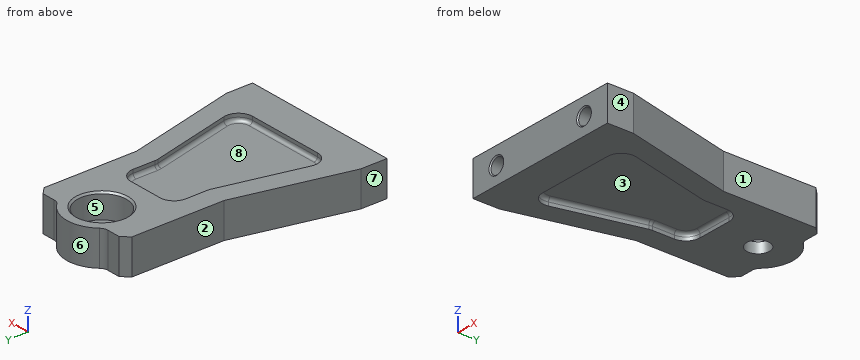
```python
from build123d import *

# Parameters (mm, degrees)
SKETCH1_R                         = 6.5
BOSS_EXTRUDE1_DEPTH               = 10
SKETCH2_R                         = 14
CUT_EXTRUDE1_DEPTH                = 14
CHAMFER1_SIZE                     = 1
CHAMFER2_SIZE                     = 4
FILLET1_R                         = 5
CUT_EXTRUDE2_DEPTH                = 4
FILLET2_R                         = 2
FILLET2_OF_MIRROR1_R              = 2
M10X1_25_TAPPED_HOLE2_D           = 8.8
M10X1_25_TAPPED_HOLE2_DEPTH       = 20
M10X1_25_TAPPED_HOLE2_CSINK_D     = 10.05
M10X1_25_TAPPED_HOLE2_CSINK_ANGLE = 90
M10X1_25_TAPPED_HOLE2_TIP         = 2.643786724


with BuildPart() as part:
    # Sketch1 → Boss-Extrude1 (new, symmetric)
    with BuildSketch(Plane.XY):
        with BuildLine():
            Line((-46, 0), (46, 0))
            Line((46, 0), (46, 15))
            Line((46, 15), (30, 80))
            Line((30, 80), (30, 137))
            Line((30, 137), (16, 137))
            ThreePointArc((16, 137), (0, 145), (-16, 137))
            Line((-16, 137), (-30, 137))
            Line((-30, 137), (-30, 80))
            Line((-30, 80), (-46, 15))
            Line((-46, 15), (-46, 0))
        make_face()
        with Locations((0, 125)):
            Circle(SKETCH1_R, mode=Mode.SUBTRACT)
    extrude(amount=BOSS_EXTRUDE1_DEPTH, both=True)

    # Sketch2 → Cut-Extrude1 (cut)
    with BuildSketch(Plane.XY.offset(10)):
        with Locations((0, 125)):
            Circle(SKETCH2_R)
    extrude(amount=-CUT_EXTRUDE1_DEPTH, mode=Mode.SUBTRACT)

    # Chamfer1
    chamfer1_edges = [part.edges().sort_by_distance(p)[0] for p in [
        (-14, 125, 10),
    ]]
    chamfer(chamfer1_edges, length=CHAMFER1_SIZE)

    # Chamfer2
    chamfer2_edges = [part.edges().sort_by_distance(p)[0] for p in [
        (-30, 137, 0),
        (30, 137, 0),
    ]]
    chamfer(chamfer2_edges, length=CHAMFER2_SIZE)

    # Fillet1
    fillet1_edges = [part.edges().sort_by_distance(p)[0] for p in [
        (-16, 137, 0),
        (16, 137, 0),
    ]]
    fillet(fillet1_edges, radius=FILLET1_R)

    # Sketch3 → Cut-Extrude2 (cut)
    with BuildSketch(Plane.XY.offset(10)):
        with BuildLine():
            Line((-18, 92), (-18, 79.514932029))
            ThreePointArc((-18, 79.514932029), (-18.058181812, 78.55185162), (-18.231880969, 77.602779652))
            Line((-18.231880969, 77.602779652), (-29.971112298, 29.912152377))
            ThreePointArc((-29.971112298, 29.912152377), (-28.49970745, 23.065287193), (-22.202993266, 20))
            Line((-22.202993266, 20), (22.202993266, 20))
            ThreePointArc((22.202993266, 20), (28.49970745, 23.065287193), (29.971112298, 29.912152377))
            Line((29.971112298, 29.912152377), (18.231880969, 77.602779652))
            ThreePointArc((18.231880969, 77.602779652), (18.058181812, 78.55185162), (18, 79.514932029))
            Line((18, 79.514932029), (18, 92))
            ThreePointArc((18, 92), (15.656854249, 97.656854249), (10, 100))
            Line((10, 100), (-10, 100))
            ThreePointArc((-10, 100), (-15.656854249, 97.656854249), (-18, 92))
        make_face()
    cut_extrude2 = extrude(amount=-CUT_EXTRUDE2_DEPTH, mode=Mode.SUBTRACT)

    # Fillet2
    fillet2_edges = [part.edges().sort_by_distance(p)[0] for p in [
        (18.058181812, 78.55185162, 6),
        (24.101496633, 53.757466014, 6),
        (28.49970745, 23.065287193, 6),
        (0, 20, 6),
        (-28.49970745, 23.065287193, 6),
        (-24.101496633, 53.757466014, 6),
        (-18.058181812, 78.55185162, 6),
        (-18, 85.757466014, 6),
        (-15.656854249, 97.656854249, 6),
        (0, 100, 6),
        (15.656854249, 97.656854249, 6),
        (18, 85.757466014, 6),
    ]]
    fillet(fillet2_edges, radius=FILLET2_R)

    # Mirror1: Cut-Extrude2 across plane
    add(cut_extrude2.mirror(Plane.XY), mode=Mode.SUBTRACT)

    # Fillet2 of Mirror1
    fillet2_of_mirror1_edges = [part.edges().sort_by_distance(p)[0] for p in [
        (18.058181812, 78.55185162, -6),
        (24.101496633, 53.757466014, -6),
        (28.49970745, 23.065287193, -6),
        (0, 20, -6),
        (-28.49970745, 23.065287193, -6),
        (-24.101496633, 53.757466014, -6),
        (-18.058181812, 78.55185162, -6),
        (-18, 85.757466014, -6),
        (-15.656854249, 97.656854249, -6),
        (0, 100, -6),
        (15.656854249, 97.656854249, -6),
        (18, 85.757466014, -6),
    ]]
    fillet(fillet2_of_mirror1_edges, radius=FILLET2_OF_MIRROR1_R)

    # M10x1.25 Tapped Hole2
    with Locations(Plane(origin=(0, 0, 0), x_dir=(-1, 0, 0), z_dir=(0, -1, 0))):
        with Locations((-30, 0), (30, 0)):
            CounterSinkHole(M10X1_25_TAPPED_HOLE2_D / 2, M10X1_25_TAPPED_HOLE2_CSINK_D / 2, depth=M10X1_25_TAPPED_HOLE2_DEPTH, counter_sink_angle=M10X1_25_TAPPED_HOLE2_CSINK_ANGLE)
            with Locations((0, 0, -(M10X1_25_TAPPED_HOLE2_DEPTH + M10X1_25_TAPPED_HOLE2_TIP / 2))):  # 118° drill point
                Cone(0, M10X1_25_TAPPED_HOLE2_D / 2, M10X1_25_TAPPED_HOLE2_TIP, mode=Mode.SUBTRACT)


solid = part.part
```
Read the model definition and answer for the solid it produces. Units are mm, in the model's axes. Face numbers are marked on the shaded views. A direction names the side the tool comes from. Round coordinates to 2 decimals unless told otherwise and drop trailing zeros. Write each loop counter-clockwise with the first axis right and the second up, starting at its lowest first coordinate (ties: lowest second). Pieces come first, ordered by that corner, then holes. Notation, with made-up numbers: (-30, 72) - (1, 72) arc R19 ccw to (1, 103) - close; hole circle Ø10 at (-38, 15.25). An arc over 180 degrees is marked (long way). One line per item, written item: value.
Q1. Find section B-B (y = 125). Determine the outline of the cut face in (x, z), and give its area (3 significant figures).
The answers:
outline: (-30, -10) - (-6.5, -10) - (-6.5, -4) - (-14, -4) - (-14, 9) - (-15, 10) - (-30, 10) - close; (6.5, -10) - (30, -10) - (30, 10) - (15, 10) - (14, 9) - (14, -4) - (6.5, -4) - close
area: 729 mm2
Q2. Each of these flat-tipped pins is pushed along its axis until it touches: P1, Ø22.5, axis at x = 0, y = 125, coming from the +Z side; P2, Ø8, axis at x = -30, z = 0, coming from the -Y side; P3, Ø12, axis at x = -35, z = 3.5, coming from the +Y side. Where does it stop, or does it pass through?
The answers:
P1: stops at z = -4
P2: stops at y = 20.24
P3: stops at y = 134
Q3. Straight lines are drawn through the part: line 1 (X direction, y = 89, z = 9.25); line 2 (Y direction, x = 0, z = 2.75); line 3 (Z direction, x = 30, y = 7.5). For each, find the intervals that lie inside material, in ascending order. Write a range as from..to.
The answers:
line 1: x = -30..-18, 18..30
line 2: y = 0..111, 139..145
line 3: z = -10..-4.4, 4.4..10
Q4. Find section D-D (x = -39.5). Determine the outline of the cut face in (y, z).
The answers:
outline: (0, -10) - (41.41, -10) - (41.41, 10) - (0, 10) - close
Q5. Find section C-C (y = 81.5). Determine the outline of the cut face in (x, z).
The answers:
outline: (-30, -10) - (-18, -10) - (-18, -8) arc R2 cw to (-16, -6) - (16, -6) arc R2 cw to (18, -8) - (18, -10) - (30, -10) - (30, 10) - (18, 10) - (18, 8) arc R2 cw to (16, 6) - (-16, 6) arc R2 cw to (-18, 8) - (-18, 10) - (-30, 10) - close
Q6. Which of the six approach directions +Z, -Z, +X, -X, +Y, -Y give full straight-line access (tool end or side, diameter ignored) to the marked faces 1, 2, 3, 4 and 5?
The answers:
face 1: +Z, -Z, +X, +Y
face 2: +Z, -Z, -X, +Y
face 3: -Z
face 4: +Z, -Z, +X, +Y, -Y
face 5: +Z
Q7. Find section A-A (x = 0). Determine the outline of the cut face in (y, z).
The answers:
outline: (0, -10) - (20, -10) - (20, -8) arc R2 cw to (22, -6) - (98, -6) arc R2 cw to (100, -8) - (100, -10) - (118.5, -10) - (118.5, -4) - (111, -4) - (111, 9) - (110, 10) - (100, 10) - (100, 8) arc R2 cw to (98, 6) - (22, 6) arc R2 cw to (20, 8) - (20, 10) - (0, 10) - close; (131.5, -10) - (145, -10) - (145, 10) - (140, 10) - (139, 9) - (139, -4) - (131.5, -4) - close
Q8. For a pull along Y with two mould halves and no side action, classify the marked faces 6, 7 and 8 as pulls with the +Y half, pulls with the -Y half, needs draft (parallel to the pull), parting line crosses it, or undercut.
The answers:
face 6: pulls with the +Y half
face 7: needs draft
face 8: undercut
